from build123d import *

# Parameters (mm, degrees)
SKETCH_1_R             = 13
EXTRUDE_2_DEPTH        = 9
SKETCH_3_W             = 860
SKETCH_3_H             = 16
EXTRUDE_3_DEPTH        = 70
SKETCH_4_W             = 140
SKETCH_4_H             = 50
EXTRUDE_5_DEPTH        = 11
SKETCH_5_R             = 13
CUT_EXTRUDE_2_DEPTH    = 903.779042734
PATTERN_LINEAR_1_COUNT = 2
PATTERN_LINEAR_1_PITCH = 80
SKETCH_6_W             = 140
SKETCH_6_H             = 50
EXTRUDE_6_DEPTH        = 6
SKETCH_7_R             = 13
CUT_EXTRUDE_3_DEPTH    = 905.248306606
PATTERN_LINEAR_2_COUNT = 2
PATTERN_LINEAR_2_PITCH = 80
SKETCH_10_W            = 429
SKETCH_10_H            = 16
EXTRUDE_8_DEPTH        = 79
EXTRUDE_9_DEPTH        = 9
SKETCH_12_W            = 140
SKETCH_12_H            = 50
EXTRUDE_10_DEPTH       = 27


with BuildPart() as part:
    # 草图1 → 凸台-拉伸2 (new body)
    with BuildSketch(Plane.XY):
        Polygon((0, 0), (860, 0), (860, 16), (804.5, 16), (804.5, 290), (724.5, 290), (644.5, 210), (644.5, 226), (215.5, 226), (215.5, 210), (135.5, 290), (55.5, 290), (55.5, 16), (0, 16), align=None)
        with Locations((95.5, 90)):
            Circle(SKETCH_1_R, mode=Mode.SUBTRACT)
        with Locations((95.5, 170)):
            Circle(SKETCH_1_R, mode=Mode.SUBTRACT)
        with Locations((95.5, 250)):
            Circle(SKETCH_1_R, mode=Mode.SUBTRACT)
        with Locations((764.5, 90)):
            Circle(SKETCH_1_R, mode=Mode.SUBTRACT)
        with Locations((764.5, 170)):
            Circle(SKETCH_1_R, mode=Mode.SUBTRACT)
        with Locations((764.5, 250)):
            Circle(SKETCH_1_R, mode=Mode.SUBTRACT)
    extrude(amount=EXTRUDE_2_DEPTH)

    # 草图3 → 凸台-拉伸3 (add)
    with BuildSketch(Plane.XY.offset(9)):
        with Locations((430, 8)):
            Rectangle(SKETCH_3_W, SKETCH_3_H)
    extrude(amount=EXTRUDE_3_DEPTH)

    # 草图4 → 凸台-拉伸5 (add)
    with BuildSketch(Plane(origin=(0, 16, 0), x_dir=(1, 0, 0), z_dir=(0, 1, 0))):
        with Locations((90, -48)):
            Rectangle(SKETCH_4_W, SKETCH_4_H)
    extrude(amount=EXTRUDE_5_DEPTH)

    # 草图5 → 切除-拉伸2 (cut, through all)
    with BuildSketch(Plane(origin=(0, 27, 0), x_dir=(1, 0, 0), z_dir=(0, 1, 0))):
        with Locations(Location((40, -48, 0), (0, 0, 270))):
            Circle(SKETCH_5_R)
    cut_extrude_2 = extrude(amount=-CUT_EXTRUDE_2_DEPTH, mode=Mode.SUBTRACT)

    # 阵列(线性)1: 切除-拉伸2 ×2
    with Locations(*[(i * PATTERN_LINEAR_1_PITCH, 0, 0) for i in range(1, PATTERN_LINEAR_1_COUNT)]):
        add(cut_extrude_2, mode=Mode.SUBTRACT)

    # 草图6 → 凸台-拉伸6 (add)
    with BuildSketch(Plane(origin=(0, 16, 0), x_dir=(1, 0, 0), z_dir=(0, 1, 0))):
        with Locations((770, -48)):
            Rectangle(SKETCH_6_W, SKETCH_6_H)
    extrude(amount=EXTRUDE_6_DEPTH)

    # 草图7 → 切除-拉伸3 (cut, through all)
    with BuildSketch(Plane(origin=(0, 22, 0), x_dir=(1, 0, 0), z_dir=(0, 1, 0))):
        with Locations(Location((820, -48, 0), (0, 0, 270))):
            Circle(SKETCH_7_R)
    cut_extrude_3 = extrude(amount=-CUT_EXTRUDE_3_DEPTH, mode=Mode.SUBTRACT)

    # 阵列(线性)2: 切除-拉伸3 ×2
    with Locations(*[(-i * PATTERN_LINEAR_2_PITCH, 0, 0) for i in range(1, PATTERN_LINEAR_2_COUNT)]):
        add(cut_extrude_3, mode=Mode.SUBTRACT)

    # 草图10 → 凸台-拉伸8 (add)
    with BuildSketch(Plane.XY.offset(9)):
        with Locations((430, 218)):
            Rectangle(SKETCH_10_W, SKETCH_10_H)
    extrude(amount=EXTRUDE_8_DEPTH)

    # 草图11 → 凸台-拉伸9 (add)
    with BuildSketch(Plane.XY.offset(9)):
        Polygon((55.5, 290), (135.5, 290), (215.5, 210), (644.5, 210), (724.5, 290), (804.5, 290), (804.5, 16), (55.5, 16), align=None)
    extrude(amount=-EXTRUDE_9_DEPTH)

    # 草图12 → 凸台-拉伸10 (add)
    with BuildSketch(Plane(origin=(0, 27, 0), x_dir=(1, 0, 0), z_dir=(0, 1, 0))):
        with Locations((90, -48)):
            Rectangle(SKETCH_12_W, SKETCH_12_H)
        with Locations((770, -48)):
            Rectangle(SKETCH_12_W, SKETCH_12_H)
    extrude(amount=-EXTRUDE_10_DEPTH)


solid = part.part
Geometry check sheet. Reference: the model listing, model coordinates, mm. A direction names the side the tool comes from. Coordinates: 2 decimals unless noted, no trailing zeros. Loops run counter-clockwise (first coordinate to the right, second up) from the corner with the lowest first, then second, coordinate; pieces in that order, holes last. Notation, with made-up numbers: (-23, 40) - (3, 40) arc R6 ccw to (3, 44) - close; hole circle Ø6 at (77, 69). An arc over 180 degrees is marked (long way). Use one line per item in the form item = value. Start each with the question number.
Item 1: Gauge pin test, flat ends, axial feed: pin 1 (12 mm diameter, centred on x = 673.5, y = 197.5, fed in from -Z); pin 2 (17.5 mm diameter, centred on y = 216.5, z = 29, fed in from +X); pin 3 (10 mm diameter, centred on y = 114, z = 2.5, fed in from -X); pin 4 (1.5 mm diameter, centred on x = 359, y = 181, fed in from +Z). Record the tip position at first contact, or that the pin passes through.
Item 2: Section check A-A, the plane z = 36. Enter the section's corners in (x, y).
Item 3: Section check D-D, the plane x = 194.5. Enter the section's corners in (y, z).
Item 4: Section check C-C, the plane y = 121. Enter the section's corners in (x, z).
Item 5: Tool access check on faces 4 (the face through (89, 27, 48)), 5 (the face through (860, 8, 39)), 6 (the face through (685.1, 250.6, 4.4)), 7 (the face through (424, 16, 39)), 8 (the face through (424, 8, 79)). Record the directions out of +Z, -Z, +X, -X, +Y, -Y that give a thin tool (end or side, any length) a straight path to the whole face; none if there is none.
Item 6: Thickness scan on probe 1 along Y at (x, z) = (263.5, 65); probe 2 along X at (y, z) = (19, 68); probe 3 along Z at (x, y) = (603, 197.5). Record the ranges inside material, lowest first.
Item 7: Section check B-B, the plane x = 576. Enter the section's corners in (y, z), and give its area (3 significant figures).
Item 8: Mould release check, pull along X, two halves, no side actions. Record for faces 1 (the face through (427, 210, 48)), 2 (the face through (176.1, 249.4, 4.4)), 3 (the face through (0, 8, 39)): +X half, -X half, draft (parallel to the pull), parting line (faces both ways), or undercut.
Computed:
q1.pin_1 = 0
q1.pin_2 = 644.5
q1.pin_3 = 55.5
q1.pin_4 = 9
q2.outline = (0, 0) - (860, 0) - (860, 16) - (840, 16) - (840, 27) - (700, 27) - (700, 16) - (160, 16) - (160, 27) - (20, 27) - (20, 16) - (0, 16) - close; (215.5, 210) - (644.5, 210) - (644.5, 226) - (215.5, 226) - close
q3.outline = (0, 0) - (231, 0) - (231, 9) - (16, 9) - (16, 79) - (0, 79) - close
q4.outline = (55.5, 0) - (804.5, 0) - (804.5, 9) - (55.5, 9) - close
q5.face_4 = +Z, +X, -X, +Y
q5.face_5 = +Z, -Z, +X, +Y, -Y
q5.face_6 = +Z, -Z, +Y
q5.face_7 = none
q5.face_8 = +Z, +X, -X, -Y
q6.probe_1 = 0 to 16, 210 to 226
q6.probe_2 = 20 to 160, 700 to 840
q6.probe_3 = 0 to 9
q7.outline = (0, 0) - (226, 0) - (226, 88) - (210, 88) - (210, 9) - (16, 9) - (16, 79) - (0, 79) - close
q7.area = 4,420 mm2
q8.face_1 = draft
q8.face_2 = undercut
q8.face_3 = -X half
